Job drawing, mm, ordinate dimensions from the low corner. One solid piece. A direction names the side the tool comes from. Coordinates: 2 decimals unless noted, no trailing zeros. Write each loop counter-clockwise with the first axis right and the second up, starting at its lowest first coordinate (ties: lowest second). Pieces come first, ordered by that corner, then holes. Notation, with made-up numbers: (45.25, 45.5) - (56.25, 45.5) arc R15 cw to (56.25, 57.5) - close; hole circle Ø2 at (89, -24.5). An arc over 180 degrees is marked (long way). Use a Markdown table: item, result.
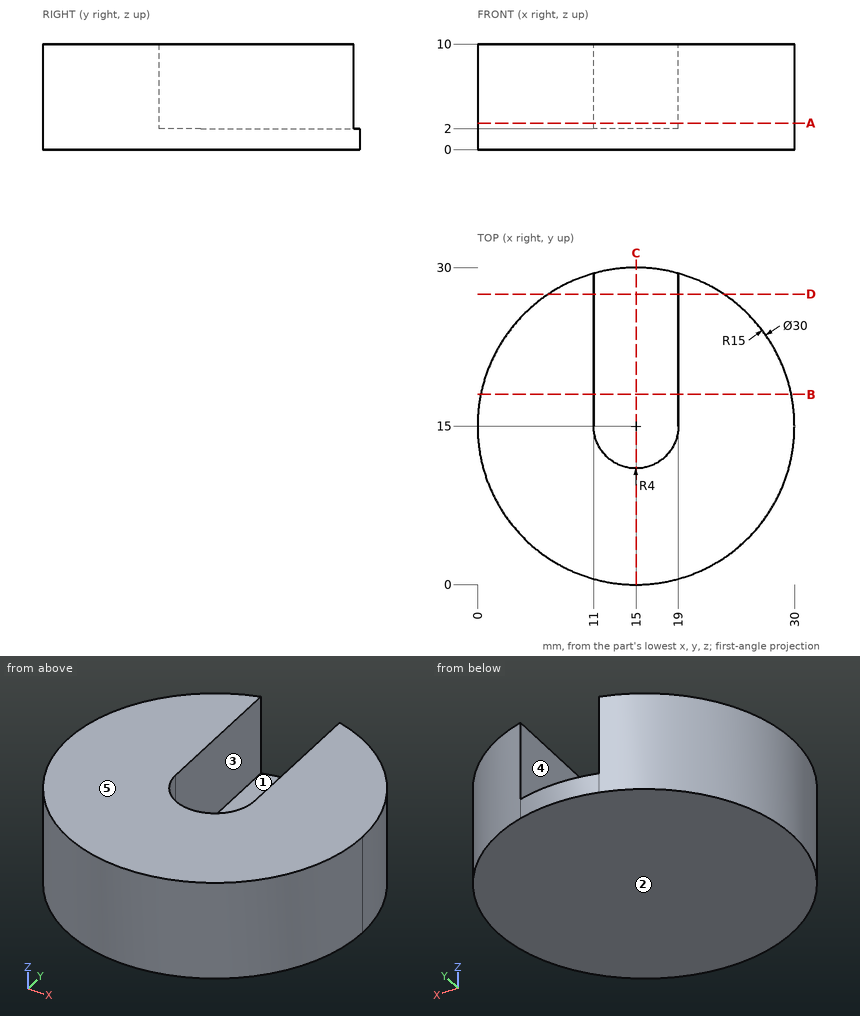
Item 1: Drill centre lines: probe 1 along X at (y, z) = (16.75, 6.5); probe 2 along X at (y, z) = (26, 5.5); probe 3 along Z at (x, y) = (13, 24.75). Where is each one in solid material? Low to high.
From the geometry:
| item | result |
|---|---|
| probe 1 | 0.1 to 11, 19 to 29.9 |
| probe 2 | 4.8 to 11, 19 to 25.2 |
| probe 3 | 0 to 2 |
Item 2: Band-saw the part on B-B, the plane y = 18. Give the cut face in (x, z), then the cut area to 3 significant figures.
From the geometry:
| item | result |
|---|---|
| outline | (0.3, 0) - (29.7, 0) - (29.7, 10) - (19, 10) - (19, 2) - (11, 2) - (11, 10) - (0.3, 10) - close |
| area | 230 mm^2 |
Item 3: Drop flat-ended pins along their axis: P1, Ø2, axis at y = 10.5, z = 8, coming from the -X side; P2, Ø1.5, axis at x = 4, z = 6.5, coming from the +Y side; P3, Ø2.5, axis at x = 16, y = 23.5, coming from the +Z side. Give the stop position or say it passes through.
From the geometry:
| item | result |
|---|---|
| P1 | x = 0.41 |
| P2 | y = 25.95 |
| P3 | z = 2 |
Item 4: Two-plate mould, pull along X, no slides. Class the marked faces 1, 2 and 3: pulls with the +X half, pulls with the -X half, needs draft (parallel to the pull), parting line crosses it, or undercut.
From the geometry:
| item | result |
|---|---|
| face 1 | undercut |
| face 2 | needs draft |
| face 3 | undercut |
Item 5: Band-saw the part on C-C, the plane x = 15. Give the cut face in (y, z), then the cut area to 3 significant figures.
From the geometry:
| item | result |
|---|---|
| outline | (0, 0) - (30, 0) - (30, 2) - (11, 2) - (11, 10) - (0, 10) - close |
| area | 148 mm^2 |
Item 6: Band-saw the part on A-A, the plane z = 2.5. Give the cut face in (x, y), then the cut area to 3 significant figures.
From the geometry:
| item | result |
|---|---|
| outline | (11, 15) - (11, 29.46) arc R15 ccw (long way) to (19, 29.46) - (19, 15) arc R4 cw to start |
| area | 563 mm^2 |
Item 7: Band-saw the part on D-D, the plane y = 27.5. Give the cut face in (x, z).
From the geometry:
| item | result |
|---|---|
| outline | (6.71, 0) - (23.29, 0) - (23.29, 10) - (19, 10) - (19, 2) - (11, 2) - (11, 10) - (6.71, 10) - close |
Item 8: Which spindle directions (+Z, -Z, +X, -X, +Y, -Y) get a long thin tool onto all of the face, cutting with end or side? Do the marked faces 4 and 5. Say none if no direction does.
From the geometry:
| item | result |
|---|---|
| face 4 | +Z, +Y |
| face 5 | +Z, +X, -X, +Y, -Y |
